from build123d import *

# Parameters (mm, degrees)
F1_DEPTH = 60
F3_DEPTH = 60.001
F5_DEPTH = 100.001


with BuildPart() as f1:
    # F0 (on Top) → F1 (new body)
    with BuildSketch(Plane.XY):
        Polygon((0, 60), (0, 0), (20, 0), (20, 15), (55, 15), (55, 0), (70, 0), (70, 20), (100, 20), (100, 60), align=None)
    extrude(amount=F1_DEPTH)

    # F2 (on Front) → F3 (cut, through all)
    with BuildSketch(Plane.XZ):
        Polygon((0, 60), (0, 40), (20, 40), (40, 60), align=None)
        Polygon((100, 60), (75, 60), (100, 35), align=None)
    extrude(amount=-F3_DEPTH, mode=Mode.SUBTRACT)

    # F4 (on face) → F5 (cut, through all)
    with BuildSketch(Plane.YZ.offset(100)):
        Polygon((0, 5), (50, 60), (0, 60), align=None)
    extrude(amount=-F5_DEPTH, mode=Mode.SUBTRACT)


solid = f1.part
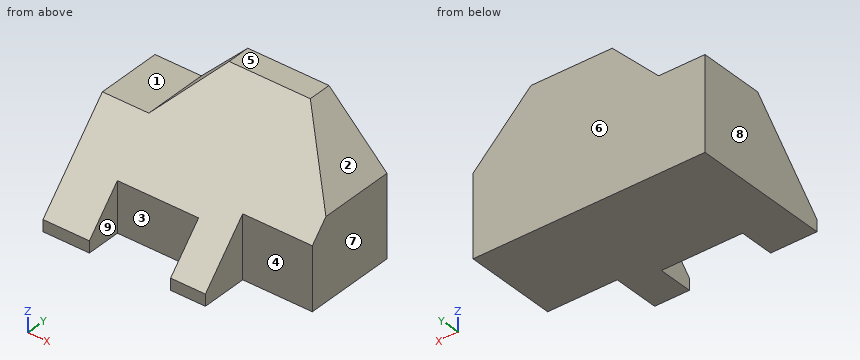
Work out the finished part from the listing and answer in its coordinate system (mm). Face numbers are marked on the shaded views. A direction names the side the tool comes from. Give positions to 0.01 mm unless a question says otherwise; leave off trailing zeros. Loops run counter-clockwise (first coordinate to the right, second up) from the corner with the lowest first, then second, coordinate; pieces in that order, holes last. Notation, with made-up numbers: (53, 52) - (73, 52) arc R23 cw to (73, 64) - close; hole circle Ø2 at (53.5, 80.5). An arc over 180 degrees is marked (long way). Answer in a Markdown table with one row per item. Add a question column.
Q1. The part is cut by section A-A (y = 34.5). Determine the outline of the cut face in (x, z), and give its area (3 significant figures).
Q2. The part is cut by section C-C (x = 42). Determine the outline of the cut face in (y, z).
Q3. Determine the mould class of the marked faces 6, 7, 8 and 9 for opening direction X: released by +X, released by -X, zero draft, split by the parting line, or undercut.
Q4. A tool of negligible diameter and unlimited length cuts with its end or side. For the marked faces 1, 2, 3, 4 and 5, from which of +Z, -Z, +X, -X, +Y, -Y can it reach the whole face along a straight path? Write none if from no direction.
Q5. The part is cut by section D-D (y = 48). Determine the outline of the cut face in (x, z), and give its area (3 significant figures).
Q6. Consider line 1 along Y through (x, z) = (78, 7.5); line 2 along Y through (x, z) = (24, 18); line 3 along Z through (x, y) = (22, 36). Determine where each line is inside the solid, lowest interval first.
Q7. Each of these flat-tipped pins is pushed along its axis until it touches: P1, Ø22, axis at x = 14.5, y = 50, coming from the +Z side; P2, Ø12, axis at y = 10, z = 10, coming from the +X side; P3, Ø8, axis at x = 40.5, y = 25.5, coming from the -Z side; P4, Ø4, axis at x = 84.5, y = 42.5, coming from the +Z side. Where does it stop, or does it pass through?
Q8. The part is cut by section B-B (y = 12.5). Determine the outline of the cut face in (x, z).
Solution:
| question | item | result |
|---|---|---|
| 1 | outline | (0, 0) - (100, 0) - (100, 35) - (92.05, 42.95) - (22.95, 42.95) - (20, 40) - (0, 40) - close |
| 1 | area | 4,200 mm² |
| 2 | outline | (15, 0) - (60, 0) - (60, 60) - (50, 60) - (15, 21.5) - close |
| 3 | face 6 | zero draft |
| 3 | face 7 | released by +X |
| 3 | face 8 | released by -X |
| 3 | face 9 | undercut |
| 4 | face 1 | +Z, -X, +Y, -Y |
| 4 | face 2 | +Z, +X, +Y, -Y |
| 4 | face 3 | +Z, -Z, -Y |
| 4 | face 4 | +Z, -Z, +X, -Y |
| 4 | face 5 | +Z, +X, -X, +Y, -Y |
| 5 | outline | (0, 0) - (100, 0) - (100, 35) - (77.2, 57.8) - (37.8, 57.8) - (20, 40) - (0, 40) - close |
| 5 | area | 5,010 mm² |
| 6 | line 1 | y = 20 to 60 |
| 6 | line 2 | y = 15 to 60 |
| 6 | line 3 | z = 0 to 42 |
| 7 | P1 | stops at z = 45.5 |
| 7 | P2 | stops at x = 70 |
| 7 | P3 | stops at z = 0 |
| 7 | P4 | stops at z = 52.41 |
| 8 | outline | (0, 0) - (20, 0) - (20, 18.75) - (0, 18.75) - close; (55, 0) - (70, 0) - (70, 18.75) - (55, 18.75) - close |
